from build123d import *

# Parameters (mm, degrees)
SKETCH1_W                       = 9.525
SKETCH1_H                       = 76.2
BOSS_EXTRUDE1_DEPTH             = 1.5875
CHAMFER2_SIZE                   = 1.5875
F_97_0_0825_DIAMETER_HOLE1_D    = 2.0955
SKETCH5_R                       = 2.38125
SKETCH5_R_2                     = 1.04775
BOSS_EXTRUDE2_DEPTH             = 3.175
BOSS_EXTRUDE4_REACH             = 77.644
SKETCH7_W                       = 1.5875
SKETCH7_H                       = 75.318017262
BOSS_EXTRUDE4_DIRECTION_2_DEPTH = 12.7
CUT_EXTRUDE1_DEPTH              = 83.855524788


with BuildPart() as part:
    # Sketch1 → Boss-Extrude1 (new body)
    with BuildSketch(Plane.XY):
        with Locations((-4.7625, 38.1)):
            Rectangle(SKETCH1_W, SKETCH1_H)
    extrude(amount=BOSS_EXTRUDE1_DEPTH)

    # Chamfer2
    chamfer2_edges = [part.edges().sort_by_distance(p)[0] for p in [
        (0, 0, 0.79375),
        (-9.525, 0, 0.79375),
        (-9.525, 76.2, 0.79375),
        (0, 76.2, 0.79375),
    ]]
    chamfer(chamfer2_edges, length=CHAMFER2_SIZE)

    # 97 _0.0825_ Diameter Hole1 (through all)
    with Locations(Plane.XY.offset(1.5875)):
        with Locations((-4.7625, 4.7625), (-4.7625, 71.4375)):
            Hole(F_97_0_0825_DIAMETER_HOLE1_D / 2)

    # Sketch5 → Boss-Extrude2 (add)
    # profile 1 of 2: a face of its own
    with BuildSketch(Plane.XY.offset(1.5875)):
        with Locations((-4.7625, 4.7625)):
            Circle(SKETCH5_R)
        with Locations((-4.7625, 4.7625)):
            Circle(SKETCH5_R_2, mode=Mode.SUBTRACT)
    # profile 2 of 2: a face of its own
    with BuildSketch(Plane.XY.offset(1.5875)):
        with Locations(Location((-4.7625, 71.4375, 0), (0, 0, 180))):
            Circle(SKETCH5_R)
        with Locations((-4.7625, 71.4375)):
            Circle(SKETCH5_R_2, mode=Mode.SUBTRACT)
    extrude(amount=BOSS_EXTRUDE2_DEPTH)

    # Boss-Extrude4: up to this face of the body (flat: up to its plane)
    boss_extrude4_end = Plane(part.part.faces().sort_by_distance((-4.7625, 38.1, 0))[0])
    # Sketch7 → Boss-Extrude4 (add, up to the picked face)
    with BuildSketch(Plane(origin=(0, 2.297711148, 13.030967461), x_dir=(-1, 0, 0), z_dir=(0, -0.1736481776669307, -0.984807753012208)), mode=Mode.PRIVATE) as boss_extrude4_sk1:
        with Locations((8.73125, 37.383342149)):
            Rectangle(SKETCH7_W, SKETCH7_H)
    boss_extrude4_tool1 = split(extrude(boss_extrude4_sk1.sketch, amount=BOSS_EXTRUDE4_REACH, mode=Mode.PRIVATE), bisect_by=boss_extrude4_end, keep=Keep.BOTH, mode=Mode.PRIVATE)
    add(boss_extrude4_tool1.solids().sort_by(Axis((-8.73125, 39.113116, 6.539418), (0, -0.1736481776669307, -0.984807753012208)))[0])

    # Sketch7 → Boss-Extrude4 direction 2 (add)
    with BuildSketch(Plane(origin=(0, 2.297711148, 13.030967461), x_dir=(-1, 0, 0), z_dir=(0, -0.1736481776669307, -0.984807753012208))):
        with Locations((8.73125, 37.383342149)):
            Rectangle(SKETCH7_W, SKETCH7_H)
    extrude(amount=-BOSS_EXTRUDE4_DIRECTION_2_DEPTH)

    # Sketch9 → Cut-Extrude1 (cut, through all)
    with BuildSketch(Plane(origin=(-7.9375, 0, 0), x_dir=(0, 0, -1), z_dir=(1, 0, 0))):
        Polygon((0, 0), (-1.5875, 0), (0, -0.279919082), align=None)
    extrude(amount=-CUT_EXTRUDE1_DEPTH, mode=Mode.SUBTRACT)


solid = part.part
For this review, take the finished solid that the model builds, in its own axes (mm). A direction names the side the tool comes from. Round coordinates to 2 decimals unless told otherwise and drop trailing zeros. Loops run counter-clockwise (first coordinate to the right, second up) from the corner with the lowest first, then second, coordinate; pieces in that order, holes last. Notation, with made-up numbers: (-31, 75) - (22, 75) arc R28 ccw to (22, 93) - close; hole circle Ø1 at (38.5, 82.25). An arc over 180 degrees is marked (long way). Use one line per item in the form item = value.
1) Mouldability with a two-part tool opening along Y and no side actions: class faces 6 (the face through (-8.72, 2.086, 13.419)), 7 (the face through (-4, 39, 1.588)), 8 (the face through (-5, 6, 4.762)) as pulls with the +Y half, pulls with the -Y half, needs draft (parallel to the pull), parting line crosses it, or undercut.
Solutions:
face_6 = pulls with the -Y half
face_7 = undercut
face_8 = needs draft
2) Wall thickness on probe 1 along Z at (x, y) = (-3.25, 53); probe 2 along X at (y, z) = (34.5, 18) (1 decimal); probe 3 along Z at (x, y) = (-6, 69.5): over which ranges is each line inside the solid? List them lowest first.
Solutions:
probe_1 = 0 to 1.59
probe_2 = -9.5 to -7.9
probe_3 = 0 to 4.76
3) We need section A-A on x = -4.5. Write out the cut boundary in (y, z), then the cut area to 3 significant figures.
Solutions:
outline = (0, 0) - (3.75, 0) - (3.75, 4.76) - (2.4, 4.76) - (2.4, 1.59) - (0, 1.59) - close; (5.78, 0) - (70.42, 0) - (70.42, 4.76) - (69.07, 4.76) - (69.07, 1.59) - (7.13, 1.59) - (7.13, 4.76) - (5.78, 4.76) - close; (72.45, 0) - (76.2, 0) - (76.2, 1.59) - (73.8, 1.59) - (73.8, 4.76) - (72.45, 4.76) - close
area = 132 mm2
4) Tool access review of faces 1 (the face through (-8.72, 41.838, 18.955)), 2 (the face through (-6, 72, 4.762)), 3 (the face through (-5, 76.2, 1)), 4 (the face through (-5.28, 2.44, 3.15)), 5 (the face through (0, 38, 1)): name each direction out of +Z, -Z, +X, -X, +Y, -Y from which nothing blocks a thin tool from reaching the whole face with its end or side.
Solutions:
face_1 = +Z, +X, -X, +Y
face_2 = +Z, +X, +Y, -Y
face_3 = +Z, -Z, +X, +Y
face_4 = +Z
face_5 = +Z, -Z, +X, +Y, -Y
5) We need section D-D on y = 16. Write out the cut boundary in (x, z) (1 decimal), then the cut area to 3 significant figures.
Solutions:
outline = (-9.5, 0) - (0, 0) - (0, 1.6) - (-7.9, 1.6) - (-7.9, 23.5) - (-9.5, 23.5) - close
area = 49.9 mm2
6) Clearance check with flat-ended pins moving along their axes: P1, Ø3, axis at y = 54, z = 7.5, coming from the +X side; P2, Ø1.3, axis at x = -4.76, y = 4.76, coming from the +Z side; P3, Ø1.4, axis at x = -6, y = 6, coming from the +Z side; P4, Ø2.5, axis at x = -5, y = 23, coming from the +Z side. State where each tip first meets the part, or that it passes through.
Solutions:
P1 = -7.94
P2 = through
P3 = 4.76
P4 = 1.59
7) We need section C-C on z = 17. Write out the cut boundary in (x, y) (1 decimal).
Solutions:
outline = (-9.5, 2.7) - (-7.9, 2.7) - (-7.9, 52.9) - (-9.5, 52.9) - close
8) We need section B-B on y = 61.5. Write out the cut boundary in (x, z) (1 decimal), then the cut area to 3 significant figures.
Solutions:
outline = (-9.5, 0) - (0, 0) - (0, 1.6) - (-7.9, 1.6) - (-7.9, 15.5) - (-9.5, 15.5) - close
area = 37.2 mm2
